Build history of the part. All positions in model axes, mm. Face numbers are marked on the shaded views. A direction names the side the tool comes from. Give positions to 0.01 mm unless a question says otherwise; leave off trailing zeros. Write each loop counter-clockwise with the first axis right and the second up, starting at its lowest first coordinate (ties: lowest second). Pieces come first, ordered by that corner, then holes.
from build123d import *

# Parameters (mm, degrees)
SKETCH1_W           = 13.97
SKETCH1_H           = 12.7
BOSS_EXTRUDE1_DEPTH = 10.16
SKETCH1_3_R         = 2.54
BOSS_EXTRUDE2_DEPTH = 17.78
BOSS_EXTRUDE3_START = 53.34
SKETCH2_R           = 3.81
BOSS_EXTRUDE3_DEPTH = 31.75
BOSS_EXTRUDE4_START = 53.34
SKETCH3_W           = 30.48
SKETCH3_H           = 6.35
BOSS_EXTRUDE4_DEPTH = 13.97
CUT_EXTRUDE1_START  = -1
SKETCH4_R           = 2.5
CUT_EXTRUDE1_DEPTH  = 87.09
SKETCH6_R           = 2.286
CUT_EXTRUDE3_DEPTH  = 18.78
SKETCH5_W           = 115.291364872
SKETCH5_H           = 73.621660508
CUT_EXTRUDE2_DEPTH  = 32.75


with BuildPart() as part:
    # Sketch1 → Boss-Extrude1 (new body, symmetric)
    with BuildSketch(Plane(origin=(0, 0, 0), x_dir=(1, 0, 0), z_dir=(0, 1, 0))):
        with Locations((60.325, 0)):
            Rectangle(SKETCH1_W, SKETCH1_H)
    boss_extrude1 = extrude(amount=BOSS_EXTRUDE1_DEPTH, both=True)

    # Sketch1_3 → Boss-Extrude2 (add, symmetric)
    with BuildSketch(Plane(origin=(0, 0, 0), x_dir=(1, 0, 0), z_dir=(0, 1, 0))):
        with Locations((57.15, 0)):
            Circle(SKETCH1_3_R)
    boss_extrude2 = extrude(amount=BOSS_EXTRUDE2_DEPTH, both=True)

    # Sketch2 → Boss-Extrude3 (add)
    with BuildSketch(Plane(origin=(0, 0, 0), x_dir=(0, 0, -1), z_dir=(1, 0, 0)).offset(BOSS_EXTRUDE3_START)):
        Circle(SKETCH2_R)
    boss_extrude3 = extrude(amount=BOSS_EXTRUDE3_DEPTH)

    # Sketch3 → Boss-Extrude4 (add)
    with BuildSketch(Plane(origin=(0, 0, 0), x_dir=(0, 0, -1), z_dir=(1, 0, 0)).offset(BOSS_EXTRUDE4_START)):
        with Locations((21.336, 4.699)):
            Rectangle(SKETCH3_W, SKETCH3_H)
        with Locations((21.336, -4.699)):
            Rectangle(SKETCH3_W, SKETCH3_H)
    boss_extrude4 = extrude(amount=BOSS_EXTRUDE4_DEPTH)

    # Sketch4 → Cut-Extrude1 (cut)
    with BuildSketch(Plane(origin=(0, 0, 0), x_dir=(0, 0, -1), z_dir=(1, 0, 0)).offset(CUT_EXTRUDE1_START)):
        Circle(SKETCH4_R)
    cut_extrude1 = extrude(amount=CUT_EXTRUDE1_DEPTH, mode=Mode.SUBTRACT)

    # Sketch6 → Cut-Extrude3 (cut, symmetric)
    with BuildSketch(Plane(origin=(0, 0, 0), x_dir=(1, 0, 0), z_dir=(0, 1, 0))):
        with Locations((57.15, 30.48)):
            Circle(SKETCH6_R)
    cut_extrude3 = extrude(amount=CUT_EXTRUDE3_DEPTH, both=True, mode=Mode.SUBTRACT)

    # Mirror11: Boss-Extrude1, Boss-Extrude2, Boss-Extrude3, Boss-Extrude4, Cut-Extrude1, Cut-Extrude3 across plane
    add(boss_extrude1.mirror(Plane(origin=(53.34, 10.16, -6.35), x_dir=(0, 0, 1), z_dir=(1, 0, 0))))
    add(boss_extrude2.mirror(Plane(origin=(53.34, 10.16, -6.35), x_dir=(0, 0, 1), z_dir=(1, 0, 0))))
    add(boss_extrude3.mirror(Plane(origin=(53.34, 10.16, -6.35), x_dir=(0, 0, 1), z_dir=(1, 0, 0))))
    add(boss_extrude4.mirror(Plane(origin=(53.34, 10.16, -6.35), x_dir=(0, 0, 1), z_dir=(1, 0, 0))))
    add(cut_extrude1.mirror(Plane(origin=(53.34, 10.16, -6.35), x_dir=(0, 0, 1), z_dir=(1, 0, 0))), mode=Mode.SUBTRACT)
    add(cut_extrude3.mirror(Plane(origin=(53.34, 10.16, -6.35), x_dir=(0, 0, 1), z_dir=(1, 0, 0))), mode=Mode.SUBTRACT)

    # Sketch5 → Cut-Extrude2 (cut, through all)
    with BuildSketch(Plane(origin=(53.34, 0, 0), x_dir=(0, 0, -1), z_dir=(1, 0, 0))):
        with Locations((14.102354185, -2.798711487)):
            Rectangle(SKETCH5_W, SKETCH5_H)
    extrude(amount=CUT_EXTRUDE2_DEPTH, mode=Mode.SUBTRACT)


solid = part.part
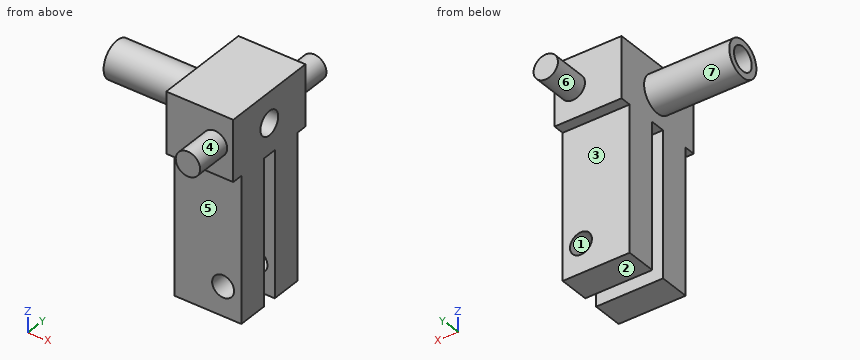
(1) Mould opens along Z. For the marked faces 1, 2 and 3 say: +Z half, -Z half, draft (parallel to the pull), parting line (faces both ways), or undercut.
(2) Saw through at A-A, the plane x = 49.53. Give the number of separate pieces and of enclosed holes in the cut face, plus the area to 3 significant figures.
(3) Saw through at C-C, the plane z = -30.48. List the corners of the cut face in (x, y).
(4) Saw through at D-D, the plane y = 0. List the corners of the cut face in (x, z).
(5) Probe line 1 (Y direction, x = 47.5, z = -14); line 2 (X direction, y = -1.5, z = -6); line 3 (X direction, y = -2.5, z = -31). List the from-to ranges inside material, lowest first.
(6) Drop flat-ended pins along their axis: pin 1 (4 mm diameter, centred on x = 48.5, z = -23.5, fed in from -Y); pin 2 (3 mm diameter, centred on x = 33, y = 5.5, fed in from +Z); pin 3 (15.5 mm diameter, centred on x = 43, z = -22, fed in from +Y); pin 4 (2.5 mm diameter, centred on x = 44, y = 9.5, fed in from -Z). Give the stop position or say it passes through.
(7) Saw through at B-B, the plane z = -15. List the corners of the cut face in (x, y).
(8) 3-axis set-ups, long thin cutter, end or side, ignore diameter. For the marked faces 4, 5, 6 and 7: which of +Z, -Z, +X, -X, +Y, -Y reach the whole face in a straight line?
Computed values:
1. face 1: undercut
1. face 2: -Z half
1. face 3: draft
2. separate pieces: 3
2. enclosed holes: 1
2. area: 642 mm2
3. outline: (39.37, -7.87) - (47.24, -7.87) - (47.24, -1.52) - (39.37, -1.52) - close; (39.37, 1.52) - (47.24, 1.52) - (47.24, 7.87) - (39.37, 7.87) - close; (51.82, -7.87) - (53.34, -7.87) - (53.34, -1.52) - (51.82, -1.52) - close; (51.82, 1.52) - (53.34, 1.52) - (53.34, 7.87) - (51.82, 7.87) - close
4. outline: (21.59, -3.81) - (39.37, -3.81) - (39.37, -6.35) - (53.34, -6.35) - (53.34, -2.5) - (21.59, -2.5) - close; (21.59, 2.5) - (53.34, 2.5) - (53.34, 6.35) - (39.37, 6.35) - (39.37, 3.81) - (21.59, 3.81) - close
5. line 1: y = -7.87 to -1.52, 1.52 to 7.87
5. line 2: x = 39.37 to 53.34
5. line 3: x = 39.37 to 47.3, 51.76 to 53.34
6. pin 1: stops at y = -7.87
6. pin 2: passes through
6. pin 3: stops at y = 7.87
6. pin 4: stops at z = -6.35
7. outline: (39.37, -7.87) - (53.34, -7.87) - (53.34, -1.52) - (39.37, -1.52) - close; (39.37, 1.52) - (53.34, 1.52) - (53.34, 7.87) - (39.37, 7.87) - close
8. face 4: -Y
8. face 5: -Z, +X, -X, -Y
8. face 6: +Y
8. face 7: -X
